CAD build for the part. Positions are in the model's coordinates, mm. A direction names the side the tool comes from. Round coordinates to 2 decimals unless told otherwise and drop trailing zeros. Write each loop counter-clockwise with the first axis right and the second up, starting at its lowest first coordinate (ties: lowest second). Pieces come first, ordered by that corner, then holes. Notation, with made-up numbers: (-24.75, -6) - (5.25, -6) arc R32 ccw to (5.25, 26) - close; hole circle Ø2 at (26, 36.25). An arc over 180 degrees is marked (long way). Use one line per item in the form item = value. Start each with the question number.
Item 1: Pin check, flat tips, straight feed: pin 1 (1.6 mm diameter, centred on x = -10, y = -52.66, fed in from +Z); pin 2 (1 mm diameter, centred on x = 8.5, z = 2.5, fed in from +Y). Stop position of each tip, or through.
Item 2: Drill centre lines: L1, parallel to Y at x = 0, z = 2.75; L2, parallel to Y at x = 6.5, z = 1.3; L3, parallel to X at y = -26, z = 0.45. Where is each one in solid material? Low to high.
Item 3: Band-saw the part on D-D, the plane y = -33. List the corners of the cut face in (x, z), and give its area (3 significant figures).
Item 4: Tool access for faces 1 (the flat face through (-15, -32, 2)), 2 (the cylindrical face through (-6.4, 5.9, 2)), 3 (the flat face through (15, -33, 2)): list every direction of +Z, -Z, +X, -X, +Y, -Y with a clear straight run to the whole face (end or side of a thin tool).
Item 5: Band-saw the part on B-B, the plane y = 0. List the corners of the cut face in (x, z).
Item 6: Band-saw the part on C-C, the plane z = 0.6. Give the number of separate pieces and of enclosed holes in the cut face, and give its area (3 significant figures).
Item 7: Band-saw the part on A-A, the plane x = 0. List the corners of the cut face in (y, z).
from build123d import *

# Parameters (mm, degrees)
CROQUIS1_R              = 1.35
CROQUIS1_R_2            = 4
CROQUIS1_R_3            = 1.25
SALIENTE_EXTRUIR1_DEPTH = 4
REDONDEO1_R             = 1.6
CROQUIS2_R              = 1
CORTAR_EXTRUIR1_DEPTH   = 4


with BuildPart() as part:
    # Croquis1 → Saliente-Extruir1 (new body)
    with BuildSketch(Plane.XY):
        with BuildLine():
            Line((-15, -10.656453444), (-15, -55.656453444))
            Line((-15, -55.656453444), (15, -55.656453444))
            Line((15, -55.656453444), (15, -10.656453444))
            ThreePointArc((15, -10.656453444), (0, 18.4), (-15, -10.656453444))
        make_face()
        with Locations((-7.071067812, -7.071067812)):
            Circle(CROQUIS1_R, mode=Mode.SUBTRACT)
        with Locations((-7.071067812, 7.071067812)):
            Circle(CROQUIS1_R, mode=Mode.SUBTRACT)
        with Locations((7.071067812, 7.071067812)):
            Circle(CROQUIS1_R, mode=Mode.SUBTRACT)
        with Locations((7.071067812, -7.071067812)):
            Circle(CROQUIS1_R, mode=Mode.SUBTRACT)
        Circle(CROQUIS1_R_2, mode=Mode.SUBTRACT)
        with Locations((-10, -52.656453444)):
            Circle(CROQUIS1_R, mode=Mode.SUBTRACT)
        with Locations(Location((10, -52.656453444, 0), (0, 0, 180))):
            Circle(CROQUIS1_R, mode=Mode.SUBTRACT)
        with Locations((9.5, -41.434010022)):
            Circle(CROQUIS1_R_3, mode=Mode.SUBTRACT)
        with Locations((-9.5, -18.434010022)):
            Circle(CROQUIS1_R_3, mode=Mode.SUBTRACT)
    extrude(amount=SALIENTE_EXTRUIR1_DEPTH)

    # Redondeo1
    redondeo1_edges = [part.edges().sort_by_distance(p)[0] for p in [
        (15, -10.656453444, 2),
        (15, -55.656453444, 2),
        (-15, -55.656453444, 2),
        (-15, -10.656453444, 2),
    ]]
    fillet(redondeo1_edges, radius=REDONDEO1_R)

    # Croquis2 → Cortar-Extruir1 (cut)
    with BuildSketch(Plane.XY.offset(4)):
        with Locations((0, -37.656453444)):
            Circle(CROQUIS2_R)
    extrude(amount=-CORTAR_EXTRUIR1_DEPTH, mode=Mode.SUBTRACT)


solid = part.part
Determined:
q1.pin_1 = through
q1.pin_2 = 16.57
q2.L1 = -55.66 to -38.66, -36.66 to -4, 4 to 18.4
q2.L2 = -55.66 to -8.29, -5.85 to 5.85, 8.29 to 17.21
q2.L3 = -15 to 15
q3.outline = (-15, 0) - (15, 0) - (15, 4) - (-15, 4) - close
q3.area = 120 mm²
q4.face_1 = +Z, -Z, -X, -Y
q4.face_2 = +Z, -Z
q4.face_3 = +Z, -Z, +X, -Y
q5.outline = (-18.4, 0) - (-4, 0) - (-4, 4) - (-18.4, 4) - close; (4, 0) - (18.4, 0) - (18.4, 4) - (4, 4) - close
q6.separate_pieces = 1
q6.enclosed_holes = 10
q6.area = 2,150 mm²
q7.outline = (-55.66, 0) - (-38.66, 0) - (-38.66, 4) - (-55.66, 4) - close; (-36.66, 0) - (-4, 0) - (-4, 4) - (-36.66, 4) - close; (4, 0) - (18.4, 0) - (18.4, 4) - (4, 4) - close
